```python
from build123d import *

# Parameters (mm, degrees)
F0_W     = 600
F0_H     = 200
F1_DEPTH = 180
F3_DEPTH = 180.001
F4_R     = 15


with BuildPart() as f1:
    # F0 (on Front) → F1 (new body)
    with BuildSketch(Plane.XZ):
        Rectangle(F0_W, F0_H)
    extrude(amount=-F1_DEPTH)

    # F2 (on face) → F3 (cut, through all)
    with BuildSketch(Plane.XZ):
        Polygon((-238.853864, -100), (-300, 100), (-300, -100), align=None)
    extrude(amount=-F3_DEPTH, mode=Mode.SUBTRACT)

    # F4
    f4_edges = [f1.edges().sort_by_distance(p)[0] for p in [
        (300, 90, 100),
        (300, 90, -100),
    ]]
    fillet(f4_edges, radius=F4_R)


solid = f1.part
```
Read the model definition and answer for the solid it produces. Units are mm, in the model's axes. Coordinates: 2 decimals unless noted, no trailing zeros. Loops run counter-clockwise (first coordinate to the right, second up) from the corner with the lowest first, then second, coordinate; pieces in that order, holes last. Notation, with made-up numbers: (83.5, -38) - (131.5, -38) arc R17 cw to (131.5, -24) - close; hole circle Ø8 at (-10.5, 32). An arc over 180 degrees is marked (long way). Answer in a Markdown table with one row per item.
1. Find section B-B, the plane z = -55. Write down the section's boundary in (x, y).
Conclusion:
| item | result |
|---|---|
| outline | (-252.61, 0) - (300, 0) - (300, 180) - (-252.61, 180) - close |
2. Given pin 1 (1 mm diameter, centred on y = 37.5, z = -34, fed in from -X), flat-ended and moving along its own axis, determine where the tip first touches the part or whether it passes through.
Conclusion:
| item | result |
|---|---|
| pin 1 | stops at x = -259.18 |
3. Find section A-A, the plane y = 115.5. Write down the section's boundary in (x, z), then the cut area to 3 significant figures.
Conclusion:
| item | result |
|---|---|
| outline | (-300, 100) - (-238.85, -100) - (285, -100) arc R15 ccw to (300, -85) - (300, 85) arc R15 ccw to (285, 100) - close |
| area | 114,000 mm² |
4. Straight lines are drawn through the part: line 1 (X direction, y = 124, z = -51); line 2 (X direction, y = 49.5, z = -26). For each, find the intervals that lie inside material, in ascending order.
Conclusion:
| item | result |
|---|---|
| line 1 | x = -253.83 to 300 |
| line 2 | x = -261.48 to 300 |
5. Find section C-C, the plane z = 5. Write down the section's boundary in (x, y).
Conclusion:
| item | result |
|---|---|
| outline | (-270.96, 0) - (300, 0) - (300, 180) - (-270.96, 180) - close |
6. Determine the mould class of faces 1 (the face through (-4, 0, 1)), 2 (the face through (-4, 180, 1)), 3 (the face through (295.72, 91.26, -95.49)) for opening direction Y: +Y half, -Y half, draft (parallel to the pull), parting line (faces both ways), or undercut.
Conclusion:
| item | result |
|---|---|
| face 1 | -Y half |
| face 2 | +Y half |
| face 3 | draft |
